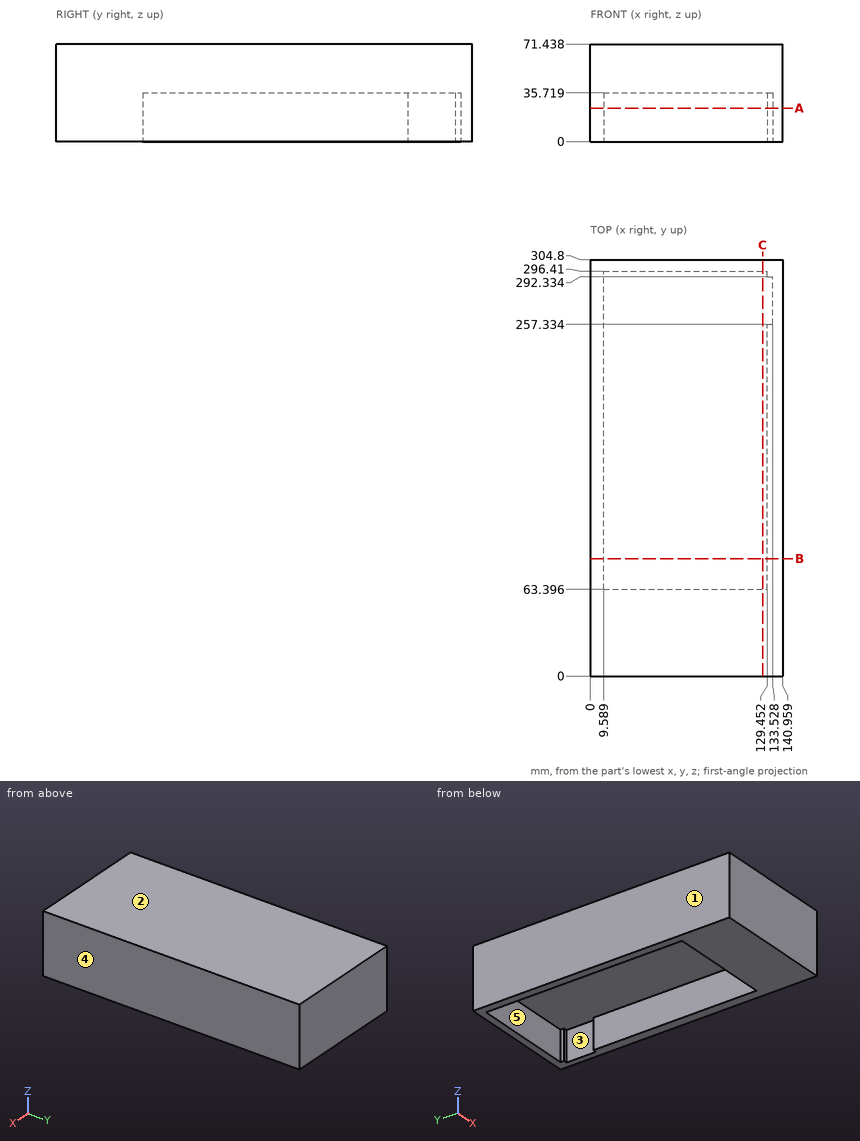
Check sheet for the drawn part. Datum: minimum x, y, z corner. Units: mm. A direction names the side the tool comes from. Round coordinates to 2 decimals unless told otherwise and drop trailing zeros. Write each loop counter-clockwise with the first axis right and the second up, starting at its lowest first coordinate (ties: lowest second). Pieces come first, ordered by that corner, then holes. Notation, with made-up numbers: (-31, 28.5) -> (19, 28.5) arc R24 ccw to (19, 49.5) -> close; hole circle Ø6 at (-23, 33). An arc over 180 degrees is marked (long way). Write each question's results on one line, items separated by ' | '. Start each with the question number.
1. Cross-section at C-C (x = 126). Enter the section's corners in (y, z) (1 decimal).
2. Material ranges on probe 1 along X at (y, z) = (76.5, 17.5); probe 2 along Y at (x, z) = (102.5, 12.5) (1 decimal); probe 3 along Y at (x, z) = (133, 31) (1 decimal), recorded low to high. Write a range as from..to.
3. Set-up check for the marked faces 4 and 5: record each of +Z, -Z, +X, -X, +Y, -Y from which the full face is reachable in a straight line by a thin tool's end or side.
4. Cross-section at A-A (z = 24.5). Enter the section's corners in (x, y) (1 decimal), then the cut area to 3 significant figures.
5. Cross-section at B-B (y = 86). Enter the section's corners in (x, z).
6. Depth check by flat-ended pin: P1, Ø2, axis at x = 43, y = 141.5, coming from the -Z side. Enter the tip coordinate at first touch or a pass-through.
7. Draft check along X on the marked faces 1, 2 and 3. Enter one of: +X half, -X half, draft (parallel to the pull), parting line (faces both ways), or undercut.
Solutions:
1) outline: (0, 0) -> (63.4, 0) -> (63.4, 35.7) -> (296.4, 35.7) -> (296.4, 0) -> (304.8, 0) -> (304.8, 71.4) -> (0, 71.4) -> close
2) probe 1: x = 0..9.59, 129.45..140.96 | probe 2: y = 0..63.4, 296.4..304.8 | probe 3: y = 0..257.3, 292.3..304.8
3) face 4: +Z, -Z, +X, +Y, -Y | face 5: -Z
4) outline: (0, 0) -> (141, 0) -> (141, 304.8) -> (0, 304.8) -> close; hole (9.6, 63.4) -> (129.5, 63.4) -> (129.5, 257.3) -> (133.5, 257.3) -> (133.5, 292.3) -> (129.5, 292.3) -> (129.5, 296.4) -> (9.6, 296.4) -> close | area: 14,900 mm2
5) outline: (0, 0) -> (9.59, 0) -> (9.59, 35.72) -> (129.45, 35.72) -> (129.45, 0) -> (140.96, 0) -> (140.96, 71.44) -> (0, 71.44) -> close
6) P1: stops at z = 35.72
7) face 1: -X half | face 2: draft | face 3: undercut
